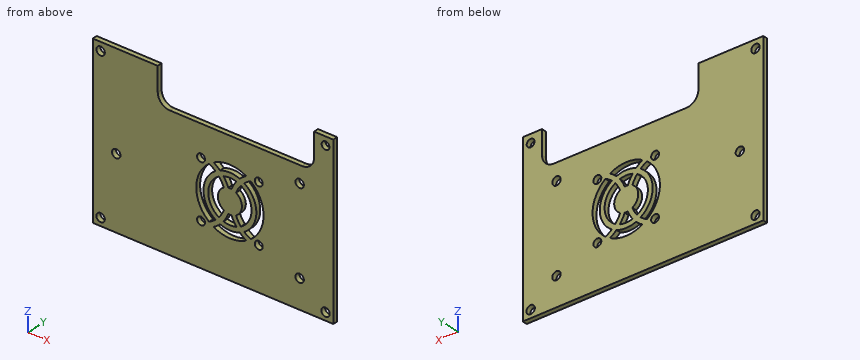
```python
from build123d import *

# Parameters (mm, degrees)
SKETCH1_W           = 100
SKETCH1_H           = 70
SKETCH1_R           = 1.75
SKETCH1_R_2         = 1.625
SKETCH1_R_3         = 14
SKETCH1_R_4         = 1.65
BOSS_EXTRUDE2_DEPTH = 2
CUT_EXTRUDE1_REACH  = 63.066
BOSS_EXTRUDE5_START = -2
BOSS_EXTRUDE5_DEPTH = 2
SKETCH11_R          = 1.75
CUT_EXTRUDE3_DEPTH  = 62.065538563


with BuildPart() as part:
    # Sketch1 → Boss-Extrude2 (new body)
    with BuildSketch(Plane(origin=(0, 0, 0), x_dir=(1, 0, 0), z_dir=(0, 1, 0))):
        Rectangle(SKETCH1_W, SKETCH1_H)
        with Locations(Location((-46.75, 31.75, 0), (0, 0, 270))):
            Circle(SKETCH1_R, mode=Mode.SUBTRACT)
        with Locations(Location((46.75, 31.75, 0), (0, 0, 90))):
            Circle(SKETCH1_R, mode=Mode.SUBTRACT)
        with Locations(Location((-46.75, -31.5, 0), (0, 0, 270))):
            Circle(SKETCH1_R, mode=Mode.SUBTRACT)
        with Locations(Location((46.75, -31.5, 0), (0, 0, 270))):
            Circle(SKETCH1_R_2, mode=Mode.SUBTRACT)
        with Locations(Location((7, 5, 0), (0, 0, 270))):
            Circle(SKETCH1_R_3, mode=Mode.SUBTRACT)
        with Locations(Location((-5, 17, 0), (0, 0, 270))):
            Circle(SKETCH1_R_4, mode=Mode.SUBTRACT)
        with Locations(Location((-5, -7, 0), (0, 0, 90))):
            Circle(SKETCH1_R_4, mode=Mode.SUBTRACT)
        with Locations(Location((19, -7, 0), (0, 0, 270))):
            Circle(SKETCH1_R_4, mode=Mode.SUBTRACT)
        with Locations(Location((19, 17, 0), (0, 0, 90))):
            Circle(SKETCH1_R_4, mode=Mode.SUBTRACT)
    extrude(amount=BOSS_EXTRUDE2_DEPTH)

    # Sketch2 → Cut-Extrude1 (cut, up to next)
    with BuildSketch(Plane(origin=(0, 2, 0), x_dir=(1, 0, 0), z_dir=(0, 1, 0)), mode=Mode.PRIVATE) as cut_extrude1_sk1:
        with BuildLine():
            Line((-18, -20), (37, -20))
            ThreePointArc((37, -20), (40.535533906, -21.464466094), (42, -25))
            Line((42, -25), (42, -35))
            Line((42, -35), (-23, -35))
            Line((-23, -35), (-23, -25))
            ThreePointArc((-23, -25), (-21.535533906, -21.464466094), (-18, -20))
        make_face()
    cut_extrude1_tool1 = extrude(cut_extrude1_sk1.sketch, amount=-CUT_EXTRUDE1_REACH, mode=Mode.PRIVATE) & part.part
    add(cut_extrude1_tool1.solids().sort_by_distance((9.5, 2, 27.57103))[0], mode=Mode.SUBTRACT)

    # Sketch3 → Boss-Extrude5 (add)
    with BuildSketch(Plane(origin=(0, 2, 0), x_dir=(1, 0, 0), z_dir=(0, 1, 0)).offset(BOSS_EXTRUDE5_START)):
        with BuildLine():
            ThreePointArc((2.907966853, -5.21054674), (7, -6), (11.092033147, -5.21054674))
            ThreePointArc((11.092033147, -5.21054674), (12.370622562, -6.311804318), (13.770604576, -7.25393462))
            ThreePointArc((13.770604576, -7.25393462), (14.740861541, -6.665293078), (15.660254038, -6))
            ThreePointArc((15.660254038, -6), (14.262684823, -5.203992902), (12.981682609, -4.231439387))
            ThreePointArc((12.981682609, -4.231439387), (18, 5), (12.981682609, 14.231439387))
            ThreePointArc((12.981682609, 14.231439387), (14.262684823, 15.203992902), (15.660254038, 16))
            ThreePointArc((15.660254038, 16), (14.740861541, 16.665293078), (13.770604576, 17.25393462))
            ThreePointArc((13.770604576, 17.25393462), (12.370622562, 16.311804318), (11.092033147, 15.21054674))
            ThreePointArc((11.092033147, 15.21054674), (7, 16), (2.907966853, 15.21054674))
            ThreePointArc((2.907966853, 15.21054674), (1.629377438, 16.311804318), (0.229395424, 17.25393462))
            ThreePointArc((0.229395424, 17.25393462), (-0.740861541, 16.665293078), (-1.660254038, 16))
            ThreePointArc((-1.660254038, 16), (-0.262684823, 15.203992902), (1.018317391, 14.231439387))
            ThreePointArc((1.018317391, 14.231439387), (-4, 5), (1.018317391, -4.231439387))
            ThreePointArc((1.018317391, -4.231439387), (-0.262684823, -5.203992902), (-1.660254038, -6))
            ThreePointArc((-1.660254038, -6), (-0.740861541, -6.665293078), (0.229395424, -7.25393462))
            ThreePointArc((0.229395424, -7.25393462), (1.629377438, -6.311804318), (2.907966853, -5.21054674))
        make_face()
        with BuildLine():
            ThreePointArc((6.336538282, 0.04421363), (7, 0), (7.663461718, 0.04421363))
            ThreePointArc((7.663461718, 0.04421363), (8.529854537, -1.849711236), (9.663461718, -3.596858244))
            ThreePointArc((9.663461718, -3.596858244), (7, -4), (4.336538282, -3.596858244))
            ThreePointArc((4.336538282, -3.596858244), (5.470145463, -1.849711236), (6.336538282, 0.04421363))
        make_face(mode=Mode.SUBTRACT)
        with BuildLine():
            ThreePointArc((4.446888819, 9.299025855), (2, 5), (4.446888819, 0.700974145))
            ThreePointArc((4.446888819, 0.700974145), (3.589514818, -1.113514772), (2.446888819, -2.763322651))
            ThreePointArc((2.446888819, -2.763322651), (-2, 5), (2.446888819, 12.763322651))
            ThreePointArc((2.446888819, 12.763322651), (3.589514818, 11.113514772), (4.446888819, 9.299025855))
        make_face(mode=Mode.SUBTRACT)
        with BuildLine():
            ThreePointArc((9.663461718, 13.596858244), (8.529854537, 11.849711236), (7.663461718, 9.95578637))
            ThreePointArc((7.663461718, 9.95578637), (7, 10), (6.336538282, 9.95578637))
            ThreePointArc((6.336538282, 9.95578637), (5.470145463, 11.849711236), (4.336538282, 13.596858244))
            ThreePointArc((4.336538282, 13.596858244), (7, 14), (9.663461718, 13.596858244))
        make_face(mode=Mode.SUBTRACT)
        with BuildLine():
            ThreePointArc((11.553111181, -2.763322651), (10.410485182, -1.113514772), (9.553111181, 0.700974145))
            ThreePointArc((9.553111181, 0.700974145), (12, 5), (9.553111181, 9.299025855))
            ThreePointArc((9.553111181, 9.299025855), (10.410485182, 11.113514772), (11.553111181, 12.763322651))
            ThreePointArc((11.553111181, 12.763322651), (16, 5), (11.553111181, -2.763322651))
        make_face(mode=Mode.SUBTRACT)
    extrude(amount=BOSS_EXTRUDE5_DEPTH)

    # Sketch11 → Cut-Extrude3 (cut, through all)
    with BuildSketch(Plane(origin=(0, 2, 0), x_dir=(1, 0, 0), z_dir=(0, 1, 0))):
        with Locations(Location((-40.25, 5, 0), (0, 0, 90))):
            Circle(SKETCH11_R)
        with Locations(Location((36, 23, 0), (0, 0, 90))):
            Circle(SKETCH11_R)
        with Locations(Location((36, -13, 0), (0, 0, 90))):
            Circle(SKETCH11_R)
    extrude(amount=-CUT_EXTRUDE3_DEPTH, mode=Mode.SUBTRACT)


solid = part.part
```
For this review, take the finished solid that the model builds, in its own axes (mm). Coordinates: 2 decimals unless noted, no trailing zeros. Loops run counter-clockwise (first coordinate to the right, second up) from the corner with the lowest first, then second, coordinate; pieces in that order, holes last. Notation, with made-up numbers: (68.25, 60.5) - (110.25, 60.5) arc R15 ccw to (110.25, 77.5) - close; hole circle Ø7 at (84, 76). An arc over 180 degrees is marked (long way). Use one line per item in the form item = value. Start each with the question number.
1) For pin 1 (4 mm diameter, centred on x = -40.25, z = -5, fed in from +Y); pin 2 (1.9 mm diameter, centred on x = 46.75, z = 31.5, fed in from +Y), all flat-tipped, find the tip position at first contact; note any pin that passes through.
2) Take a section at A-A (x = 46.75). State the section outline as (y, z) points (3 decimals).
3) Take a section at B-B (z = -31.75). State the section outline as (x, y) points.
4) To check wall thickness, follow probe 1 along Z at (x, y) = (36, 1.5); probe 2 along Z at (x, y) = (7.5, 1.6); probe 3 along X at (y, z) = (0.9, 31.5) (3 decimals). State the ranges of each line that lie inside material, in increasing order. Write a range as from..to.
5) Take a section at C-C (x = 19). State the section outline as (y, z) points.
6) Take a section at D-D (z = 13). State the section outline as (x, y) points, plus the area to 3 significant figures.
From the geometry:
q1.pin_1 = 2
q1.pin_2 = through
q2.outline = (0, -35) - (2, -35) - (2, -33.5) - (0, -33.5) - close; (0, -30) - (2, -30) - (2, 29.875) - (0, 29.875) - close; (0, 33.125) - (2, 33.125) - (2, 35) - (0, 35) - close
q3.outline = (-50, 0) - (-48.5, 0) - (-48.5, 2) - (-50, 2) - close; (-45, 0) - (45, 0) - (45, 2) - (-45, 2) - close; (48.5, 0) - (50, 0) - (50, 2) - (48.5, 2) - close
q4.probe_1 = -35..-24.75, -21.25..11.25, 14.75..20
q4.probe_2 = -35..-18.99, -15.99..-13.99, -9.97..-0.03, 3.99..5.99, 8.99..20
q4.probe_3 = -50..-48.5, -45..-23, 42..45.125, 48.375..50
q5.outline = (0, -35) - (2, -35) - (2, -18.65) - (0, -18.65) - close; (0, -15.35) - (2, -15.35) - (2, -12.21) - (0, -12.21) - close; (0, 2.21) - (2, 2.21) - (2, 5.35) - (0, 5.35) - close; (0, 8.65) - (2, 8.65) - (2, 20) - (0, 20) - close
q6.outline = (-50, 0) - (34.25, 0) - (34.25, 2) - (-50, 2) - close; (37.75, 0) - (50, 0) - (50, 2) - (37.75, 2) - close
q6.area = 193 mm2
